from build123d import *

# Parameters (mm, degrees)
SKETCH1_R           = 15.115
BOSS_EXTRUDE1_DEPTH = 20
CUT_EXTRUDE1_DEPTH  = 40.272332818
CUT_EXTRUDE3_DEPTH  = 40.272332818
SKETCH8_R           = 1.99
BOSS_EXTRUDE2_DEPTH = 65
SKETCH9_R           = 1.25
CUT_EXTRUDE4_DEPTH  = 2
SKETCH11_R          = 1.99
BOSS_EXTRUDE3_DEPTH = 96.4
SKETCH12_R          = 1.25
CUT_EXTRUDE5_DEPTH  = 2
SKETCH13_R          = 1.99
BOSS_EXTRUDE4_DEPTH = 81.15
SKETCH14_R          = 1.25
CUT_EXTRUDE6_DEPTH  = 2
SKETCH15_R          = 1.99
BOSS_EXTRUDE5_DEPTH = 60
SKETCH16_R          = 1.25
CUT_EXTRUDE7_DEPTH  = 2
SKETCH17_R          = 1.99
BOSS_EXTRUDE6_DEPTH = 60
SKETCH18_R          = 1.25
CUT_EXTRUDE8_DEPTH  = 2


with BuildPart() as part:
    # Sketch1 → Boss-Extrude1 (new body)
    with BuildSketch(Plane(origin=(0, 0, 0), x_dir=(1, 0, 0), z_dir=(0, 1, 0))):
        with Locations(Location((0, 0, 0), (0, 0, 270))):
            Circle(SKETCH1_R)
    extrude(amount=-BOSS_EXTRUDE1_DEPTH)

    # Sketch3 → Cut-Extrude1 (cut, through all)
    with BuildSketch(Plane(origin=(15.115, 0, 0), x_dir=(0, 0, -1), z_dir=(1, 0, 0))):
        Polygon((-8.905426603, 0), (-15.115, -20), (-15.115, 0), align=None)
        Polygon((4.07457383, 0), (15.115, -8.259757639), (15.115, 0), align=None)
    extrude(amount=-CUT_EXTRUDE1_DEPTH, mode=Mode.SUBTRACT)

    # Sketch7 → Cut-Extrude3 (cut, through all)
    with BuildSketch(Plane.XY.offset(15.115)):
        Polygon((15.115, 0), (9.75, 0), (15.115, -20), align=None)
        Polygon((-15.115, -20), (-15.115, 0), (-9.75, 0), align=None)
    extrude(amount=-CUT_EXTRUDE3_DEPTH, mode=Mode.SUBTRACT)

    # Sketch8 → Boss-Extrude2 (add)
    with BuildSketch(Plane(origin=(0, 0, 0), x_dir=(1, 0, 0), z_dir=(0, 1, 0))):
        with Locations(Location((-5.953992214, -5.238739903, 0), (0, 0, 270))):
            Circle(SKETCH8_R)
    extrude(amount=BOSS_EXTRUDE2_DEPTH)

    # Sketch9 → Cut-Extrude4 (cut)
    with BuildSketch(Plane(origin=(0, 65, 0), x_dir=(1, 0, 0), z_dir=(0, 1, 0))):
        with Locations(Location((-5.953992214, -5.238739903, 0), (0, 0, 270))):
            Circle(SKETCH9_R)
    extrude(amount=-CUT_EXTRUDE4_DEPTH, mode=Mode.SUBTRACT)

    # Sketch11 → Boss-Extrude3 (add)
    with BuildSketch(Plane(origin=(0, 2.521846553, 8.12244704), x_dir=(1, 0, 0), z_dir=(0, 0.296515806173068, 0.9550279455018769))):
        with Locations(Location((-4.312884214, -5.801881574, 0), (0, 0, 90))):
            Circle(SKETCH11_R)
    extrude(amount=BOSS_EXTRUDE3_DEPTH)

    # Sketch12 → Cut-Extrude5 (cut)
    with BuildSketch(Plane(origin=(0, 31.105970268, 100.187140986), x_dir=(1, 0, 0), z_dir=(0, 0.2965158061730681, 0.9550279455018768))):
        with Locations(Location((-4.312884214, -5.801881574, 0), (0, 0, 270))):
            Circle(SKETCH12_R)
    extrude(amount=-CUT_EXTRUDE5_DEPTH, mode=Mode.SUBTRACT)

    # Sketch13 → Boss-Extrude4 (add)
    with BuildSketch(Plane(origin=(9.095505077, 2.439869237, 0), x_dir=(0, 0, -1), z_dir=(0.9658531542677156, 0.25909010863231474, 0))):
        with Locations(Location((2.631146058, -5.274029077, 0), (0, 0, 270))):
            Circle(SKETCH13_R)
    extrude(amount=BOSS_EXTRUDE4_DEPTH)

    # Sketch14 → Cut-Extrude6 (cut)
    with BuildSketch(Plane(origin=(87.474488546, 23.465031552, 0), x_dir=(0, 0, -1), z_dir=(0.9658531542677156, 0.2590901086323148, 0))):
        with Locations(Location((2.631146058, -5.274029077, 0), (0, 0, 90))):
            Circle(SKETCH14_R)
    extrude(amount=-CUT_EXTRUDE6_DEPTH, mode=Mode.SUBTRACT)

    # Sketch15 → Boss-Extrude5 (add)
    with BuildSketch(Plane(origin=(-9.095505077, 2.439869237, 0), x_dir=(0, 0, 1), z_dir=(-0.9658531542677156, 0.25909010863231474, 0))):
        with Locations(Location((-2.63114606, -5.274029079, 0), (0, 0, 90))):
            Circle(SKETCH15_R)
    extrude(amount=BOSS_EXTRUDE5_DEPTH)

    # Sketch16 → Cut-Extrude7 (cut)
    with BuildSketch(Plane(origin=(-67.046694333, 17.985275755, 0), x_dir=(0, 0, 1), z_dir=(-0.9658531542677156, 0.2590901086323148, 0))):
        with Locations(Location((-2.63114606, -5.274029079, 0), (0, 0, 270))):
            Circle(SKETCH16_R)
    extrude(amount=-CUT_EXTRUDE7_DEPTH, mode=Mode.SUBTRACT)

    # Sketch17 → Boss-Extrude6 (add)
    with BuildSketch(Plane(origin=(0, 1.95442878, -1.462181603), x_dir=(1, 0, 0), z_dir=(0, 0.8007152420957264, -0.5990451577932857))):
        with Locations(Location((0, 7.441155509, 0), (0, 0, 90))):
            Circle(SKETCH17_R)
    extrude(amount=BOSS_EXTRUDE6_DEPTH)

    # Sketch18 → Cut-Extrude8 (cut)
    with BuildSketch(Plane(origin=(0, 49.997343305, -37.404891071), x_dir=(1, 0, 0), z_dir=(0, 0.8007152420957262, -0.5990451577932858))):
        with Locations(Location((0, 7.441155509, 0), (0, 0, 270))):
            Circle(SKETCH18_R)
    extrude(amount=-CUT_EXTRUDE8_DEPTH, mode=Mode.SUBTRACT)


solid = part.part
Design review of the part built by this model. Coordinates are the model's own, in mm. A direction names the side the tool comes from. Coordinates: 2 decimals unless noted, no trailing zeros. Order: outer loops, then holes, each group sorted by start corner. A loop starts at its lowest first (then second) coordinate and runs counter-clockwise, first axis right, second up. Notation, with made-up numbers: (29, 67) -> (33, 67) arc R21 cw to (33, 76) -> close; hole circle Ø6 at (-18.75, 2). An arc over 180 degrees is marked (long way). Use one line per item in the form item = value. Start each with the question number.
(1) Add section A-A on y = 56. State the section outline as (x, z) points.
(2) For faces 5 (the cylindrical face through (-39.55, 3.09, -2.72)), 6 (the flat face through (0, 0, 2)), list the 3-axis set-ups (+Z, -Z, +X, -X, +Y, -Y) from which the entire face can be reached by the end or side of a thin tool; tool diameter is ignored.
(3) Insertion check: pin 1 (1 mm diameter, centred on y = 11, z = 7.5, fed in from +X); pin 2 (10.5 mm diameter, centred on x = 1.5, z = 5.5, fed in from +Y); pin 3 (8 mm diameter, centred on y = 17.5, z = 58.5, fed in from -X). Each pin has a flat end and moves straight along its axis. Give the tip position at first contact, or say it passes through.
(4) For probe 1 along X at (y, z) = (13, -19); probe 2 along X at (y, z) = (39, 5.5); probe 3 along Z at (x, y) = (30, 1.5), list the stretches that pass through material, from the lowest coordinate up.
(5) The part is to be moulded in two halves that separate along Z. For faces 1 (the cylindrical face through (-10.727, -14.575, 10.649)), 2 (the flat face through (0, -20, 0)), 3 (the cylindrical face through (-4.4, 9.174, 55.82)), 4 (the cylindrical face through (0.33, -13.94, -15.11)), say which applies: +Z half, -Z half, draft (parallel to the pull), parting line (faces both ways), or undercut.
Answer block:
q1.outline = circle Ø3.98 at (-5.95, 5.24)
q2.face_5 = none
q2.face_6 = +Y
q3.pin_1 = -5.03
q3.pin_2 = 0
q3.pin_3 = -5.92
q4.probe_1 = -1.99 to 1.99
q4.probe_2 = -7.93 to -3.98
q4.probe_3 = -4.32 to -0.94
q5.face_1 = +Z half
q5.face_2 = draft
q5.face_3 = undercut
q5.face_4 = -Z half
